Design review of the part built by this model. Coordinates are the model's own, in mm. A direction names the side the tool comes from. Give positions to 0.01 mm unless a question says otherwise; leave off trailing zeros. Loops run counter-clockwise (first coordinate to the right, second up) from the corner with the lowest first, then second, coordinate; pieces in that order, holes last.
from build123d import *

# Parameters (mm, degrees)
BOSS_EXTRUDE1_DEPTH      = 5
BOSS_EXTRUDE1_DEPTH_BACK = 30
SKETCH1_R                = 38
SKETCH1_R_2              = 27.5
BOSS_EXTRUDE2_DEPTH      = 3
BOSS_EXTRUDE2_DEPTH_BACK = 7
SKETCH1_3_R              = 7.5
SKETCH1_4_R              = 3.5
BOSS_EXTRUDE3_DEPTH      = 50
SKETCH1_5_R              = 27.5
SKETCH1_5_R_2            = 7.5
BOSS_EXTRUDE4_DEPTH      = 1
FILLET1_R                = 5
FILLET2_R                = 1


with BuildPart() as part:
    # Sketch1 → Boss-Extrude1 (new, two sides: drawn at the far end of the back side and taken through both)
    with BuildSketch(Plane(origin=(0, 0, 0), x_dir=(0, 0, -1), z_dir=(1, 0, 0)).offset(-BOSS_EXTRUDE1_DEPTH_BACK)):
        Circle(SKETCH1_R)
        Circle(SKETCH1_R_2, mode=Mode.SUBTRACT)
    extrude(amount=BOSS_EXTRUDE1_DEPTH + BOSS_EXTRUDE1_DEPTH_BACK)



with BuildPart() as body_2:
    # Sketch1<3> → Boss-Extrude2 (new, two sides: drawn at the far end of the back side and taken through both)
    with BuildSketch(Plane(origin=(0, 0, 0), x_dir=(0, 0, -1), z_dir=(1, 0, 0)).offset(-BOSS_EXTRUDE2_DEPTH_BACK)):
        Circle(SKETCH1_3_R)
    extrude(amount=BOSS_EXTRUDE2_DEPTH + BOSS_EXTRUDE2_DEPTH_BACK)

    # Sketch1<4> → Boss-Extrude3 (add)
    with BuildSketch(Plane(origin=(0, 0, 0), x_dir=(0, 0, -1), z_dir=(1, 0, 0))):
        Circle(SKETCH1_4_R)
    extrude(amount=-BOSS_EXTRUDE3_DEPTH)


with BuildPart() as part_1:
    add(part.part)

    add(body_2.part)  # Boss-Extrude4 merges body 2
    # Sketch1<5> → Boss-Extrude4 (add, symmetric)
    with BuildSketch(Plane(origin=(0, 0, 0), x_dir=(0, 0, -1), z_dir=(1, 0, 0))):
        Circle(SKETCH1_5_R)
        Circle(SKETCH1_5_R_2, mode=Mode.SUBTRACT)
    extrude(amount=BOSS_EXTRUDE4_DEPTH, both=True)

    # Fillet1
    fillet1_edges = [part_1.edges().sort_by_distance(p)[0] for p in [
        (5, 0, 38),
        (-30, 0, 38),
    ]]
    fillet(fillet1_edges, radius=FILLET1_R - 0.0001)  # a hair under: the kernel refuses the full size

    # Fillet2
    fillet2_edges = [part_1.edges().sort_by_distance(p)[0] for p in [
        (3, 0, 7.5),
    ]]
    fillet(fillet2_edges, radius=FILLET2_R)


solid = part_1.part
Q1. Take a section at D-D (x = -31.5). Give the boundary of the cut face in (y, z).
Results:
outline: circle Ø7 at (0, 0)
Q2. Wall thickness on line 1 (Y direction, x = -18.75, z = 0); line 2 (Z direction, x = 2.5, y = 5.5); line 3 (Y direction, x = 2, z = 0): over which ranges is each line inside the solid? List them lowest first.
Results:
line 1: y = -38 to -27.5, -3.5 to 3.5, 27.5 to 38
line 2: z = -36.92 to -26.94, -4.9 to 4.9, 26.94 to 36.92
line 3: y = -37.58 to -27.5, -7.5 to 7.5, 27.5 to 37.58
Q3. Draft analysis for pull direction Z (two halves, no side actions). For faces 4 (the face through (-12.675, -33.713, -17.535)), 5 (the face through (-1, -6, -6)), 6 (the face through (5, 25, 12)), state which applies: pulls with the +Z half, pulls with the -Z half, needs draft (parallel to the pull), parting line crosses it, or undercut.
Results:
face 4: parting line crosses it
face 5: undercut
face 6: needs draft
Q4. Insertion check: pin 1 (10 mm diameter, centred on y = 17.5, z = 7, fed in from +X); pin 2 (3 mm diameter, centred on x = -6.5, z = 16.5, fed in from +Y); pin 3 (20 mm diameter, centred on y = -10, z = 7, fed in from -X); pin 4 (10 mm diameter, centred on x = -14, y = -8.5, fed in from +Z). Each pin has a flat end and moves straight along its axis. Give the tip position at first contact, or say it passes through.
Results:
pin 1: stops at x = 1
pin 2: stops at y = 34.91
pin 3: stops at x = -50
pin 4: stops at z = 37.84
Q5. Tool access review of faces 1 (the face through (-50, 0, 0)), 2 (the face through (2.972, -26.846, 5.961)), 3 (the face through (-15.703, -26.846, 5.961)): name each direction out of +Z, -Z, +X, -X, +Y, -Y from which nothing blocks a thin tool from reaching the whole face with its end or side.
Results:
face 1: +Z, -Z, -X, +Y, -Y
face 2: +X
face 3: -X
Q6. Take a section at A-A (x = -18). Give the boundary of the cut face in (y, z).
Results:
outline: circle Ø76 at (0, 0); circle Ø7 at (0, 0); hole circle Ø55 at (0, 0)
